```python
from build123d import *

# Parameters (mm, degrees)
F0_R     = 30
F1_DEPTH = 10
F2_R     = 3
F3_R     = 5
F4_DEPTH = 6
F6_W     = 36.4418011159
F6_H     = 26.4000613242
F6_R     = 5
F7_DEPTH = 4
F8_R     = 3
F9_DEPTH = 25


with BuildPart() as f1:
    # F0 (on Front) → F1 (new body)
    with BuildSketch(Plane.XZ):
        Circle(F0_R)
    extrude(amount=F1_DEPTH)

    # F2
    f2_edges = [f1.edges().sort_by_distance(p)[0] for p in [
        (30, -5, 0),
        (-30, 0, 0),
        (-30, -10, 0),
    ]]
    fillet(f2_edges, radius=F2_R)

    # F3 (on face) → F4 (join)
    with BuildSketch(Plane.XZ.offset(10)):
        Circle(F3_R)
    extrude(amount=F4_DEPTH)


with BuildPart() as f5_1:
    # F5: instance of F1
    add(f1.part.mirror(Plane.XZ.offset(16)))


with BuildPart() as f1_1:
    add(f1.part)

    add(f5_1.part)  # F7 merges F5_1
    # F6 (on face) → F7 (join, symmetric)
    with BuildSketch(Plane.XZ.offset(16)):
        with Locations((-4.939888604, -0.2429457381)):
            Rectangle(F6_W, F6_H)
        Circle(F6_R, mode=Mode.SUBTRACT)
    extrude(amount=F7_DEPTH, both=True)

    # F8 (on face) → F9 (join)
    with BuildSketch(Plane.XY.offset(12.957084924)):
        with Locations((-19.1607891619, -16)):
            Circle(F8_R)
    extrude(amount=F9_DEPTH)


solid = f1_1.part
```
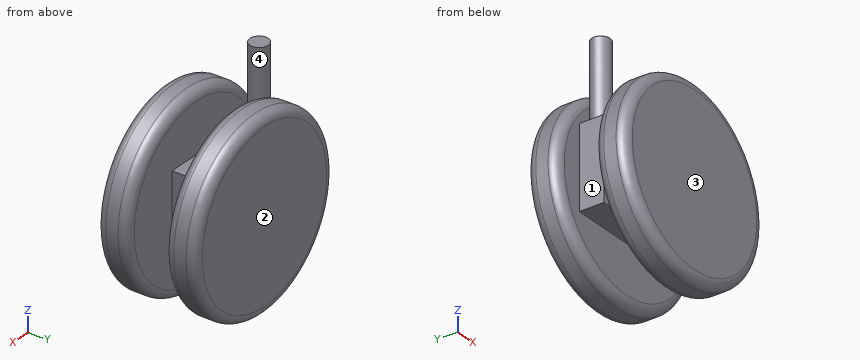
The listing builds one solid part. Answer for the finished solid, in the listing's coordinates (mm). Face numbers are marked on the shaded views. Round coordinates to 2 decimals unless told otherwise and drop trailing zeros. Write each loop counter-clockwise with the first axis right and the second up, starting at its lowest first coordinate (ties: lowest second). Pieces come first, ordered by that corner, then holes. Notation, with made-up numbers: (71.5, -31.75) -> (127.5, -31.75) arc R23 cw to (127.5, -6.75) -> close; hole circle Ø7 at (28, -36). An arc over 180 degrees is marked (long way). Answer as a JSON object with one key per item and string values. Group by question number.
Q1. Determine the mould class of the marked faces 1, 2, 3 and 4 for opening direction Y: pulls with the +Y half, pulls with the -Y half, needs draft (parallel to the pull), parting line crosses it, or undercut.
Q2. Each of these flat-tipped pins is pushed along its axis until it touches: pin 1 Ø1.5 at (x, z) = (-19.5, -21.5) entering from -Y; pin 2 Ø4 at (y, z) = (-24.5, 20.5) entering from +X; pin 3 Ø12 at (x, y) = (9.5, -13) entering from -Z; pin 4 Ø1.5 at (y, z) = (-21, -14.5) entering from +X (1 decimal). Where does it stop, or does it pass through?
Q3. Section B-B (y = -16) is taken. Write down the section's boundary in (x, z), plus the area to 3 significant figures.
Q4. Section D-D (x = -12) is taken. Count the separate pieces of the cut face and the enclosed holes in it, plus the area to 3 significant figures.
Q5. Straight lines are drawn through the part: line 1 along Y through (x, z) = (11, 11); line 2 along Y through (x, z) = (5, 26); line 3 along X through (y, z) = (-18.5, -5). For each, find the intervals that lie inside material, in ascending order.
Q6. Section A-A (x = 0) is taken. Write down the section's boundary in (y, z).
Q7. Section C-C (z = 31.5) is taken. Write down the section's boundary in (x, y).
Check values:
{
 "1": {"face 1": "undercut", "face 2": "pulls with the +Y half", "face 3": "pulls with the -Y half", "face 4": "undercut"},
 "2": {"pin 1": "y = -31.72", "pin 2": "x = 23.59", "pin 3": "z = -29.18", "pin 4": "through"},
 "3": {"outline": "(-23.16, -13.44) -> (13.28, -13.44) -> (13.28, 12.96) -> (-16.16, 12.96) -> (-16.16, 37.96) -> (-22.16, 37.96) -> (-22.16, 12.96) -> (-23.16, 12.96) -> close", "area": "1,110 mm^2"},
 "4": {"separate pieces": "3", "enclosed holes": "0", "area": "1,290 mm^2"},
 "5": {"line 1": "-32 to -22, -20 to -12, -10 to 0", "line 2": "-32 to -22, -10 to 0", "line 3": "-23.16 to 13.28"},
 "6": {"outline": "(-32, -27) arc R3 ccw to (-29, -30) -> (-25, -30) arc R3 ccw to (-22, -27) -> (-22, -5) -> (-20, -5) -> (-20, -13.44) -> (-12, -13.44) -> (-12, -5) -> (-10, -5) -> (-10, -27) arc R3 ccw to (-7, -30) -> (-3, -30) arc R3 ccw to (0, -27) -> (0, 27) arc R3 ccw to (-3, 30) -> (-7, 30) arc R3 ccw to (-10, 27) -> (-10, 5) -> (-12, 5) -> (-12, 12.96) -> (-20, 12.96) -> (-20, 5) -> (-22, 5) -> (-22, 27) arc R3 ccw to (-25, 30) -> (-29, 30) arc R3 ccw to (-32, 27) -> close"},
 "7": {"outline": "circle Ø6 at (-19.16, -16)"}
}
